Source: CAD feature listing. Evaluate the final solid. Frame: model axes, mm. Face numbers are marked on the shaded views. A direction names the side the tool comes from. Round coordinates to 2 decimals unless told otherwise and drop trailing zeros. Loops run counter-clockwise (first coordinate to the right, second up) from the corner with the lowest first, then second, coordinate; pieces in that order, holes last.
(1) Section A-A, the plane x = 12.5. Return the cut outline in (y, z).
(2) Section B-B, the plane y = 0. Return the cut outline in (x, z), plus the area to 3 significant figures.
(3) Section C-C, the plane z = 4.5. Return the cut outline in (x, y), plus the area to 3 significant figures.
(4) Set-up query: the marked faces 5 and 6. Return all of +Z, -Z, +X, -X, +Y, -Y with unobstructed straight access to the full face (end or side cutting, diameter ignored); none if empty.
(5) Section D-D, the plane x = 0. Return the cut outline in (y, z), plus the area to 3 significant figures.
(6) First-contact query: pin 1 Ø5 at (x, y) = (-2.5, 2.5) entering from +Z; pin 2 Ø2.5 at (x, y) = (24.5, -1.5) entering from +Z; pin 3 Ø1.9 at (x, y) = (-11.5, 0) entering from -Z. Flat tips, straight axial feed; report the tip coordinate or a pass-through.
(7) Mould query, pull axis X, two halves, no side actions, for the marked faces 1, 2, 3 and 4. Classes: pulls with the +X half, pulls with the -X half, needs draft (parallel to the pull), parting line crosses it, or undercut.
(8) Material intervals for probe 1 along Y at (x, z) = (0, 6.5); probe 2 along Y at (x, z) = (-11.5, 5.25); probe 3 along X at (y, z) = (1.5, 1), sorted ascending.
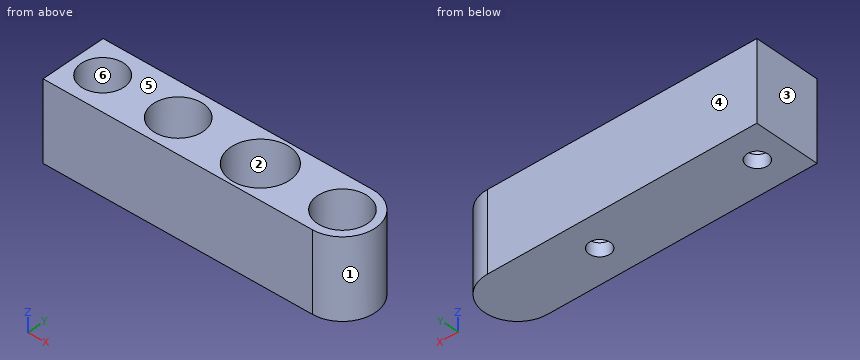
```python
from build123d import *

# Parameters (mm, degrees)
SKETCH_R     = 3.8
SKETCH_R_2   = 4.5
SKETCH_R_3   = 3.25
PAD_DEPTH    = 10
SKETCH001_R  = 1.6
PAD001_DEPTH = 2


with BuildPart() as part:
    # Sketch → Pad (new body)
    with BuildSketch(Plane.XY):
        with BuildLine():
            ThreePointArc((25, -5), (30, 0), (25, 5))
            Line((0, 5), (25, 5))
            Line((0, 5), (-16, 5))
            Line((-16, 5), (-16, -5))
            Line((-16, -5), (0, -5))
            Line((0, -5), (25, -5))
        make_face()
        Circle(SKETCH_R, mode=Mode.SUBTRACT)
        with Locations((25, 0)):
            Circle(SKETCH_R, mode=Mode.SUBTRACT)
        with Locations((12.5, 0)):
            Circle(SKETCH_R_2, mode=Mode.SUBTRACT)
        with Locations((-11.5, 0)):
            Circle(SKETCH_R_3, mode=Mode.SUBTRACT)
    extrude(amount=PAD_DEPTH)

    # Sketch001 (on Face11 of Pad) → Pad001 (join)
    with BuildSketch(Plane(origin=(0, 0, 0), x_dir=(1, 0, 0), z_dir=(0, 0, -1))):
        with BuildLine():
            ThreePointArc((25, -5), (30, 0), (25, 5))
            Line((0, 5), (25, 5))
            Line((0, 5), (-16, 5))
            Line((-16, 5), (-16, -5))
            Line((-16, -5), (0, -5))
            Line((0, -5), (25, -5))
        make_face()
        with Locations((12.5, 0)):
            Circle(SKETCH001_R, mode=Mode.SUBTRACT)
        with Locations((-11.5, 0)):
            Circle(SKETCH001_R, mode=Mode.SUBTRACT)
    extrude(amount=PAD001_DEPTH)


solid = part.part
```
Output values:
1. outline: (-5, -2) - (-1.6, -2) - (-1.6, 0) - (-4.5, 0) - (-4.5, 10) - (-5, 10) - close; (1.6, -2) - (5, -2) - (5, 10) - (4.5, 10) - (4.5, 0) - (1.6, 0) - close
2. outline: (-16, -2) - (-13.1, -2) - (-13.1, 0) - (-14.75, 0) - (-14.75, 10) - (-16, 10) - close; (-9.9, -2) - (10.9, -2) - (10.9, 0) - (8, 0) - (8, 10) - (3.8, 10) - (3.8, 0) - (-3.8, 0) - (-3.8, 10) - (-8.25, 10) - (-8.25, 0) - (-9.9, 0) - close; (14.1, -2) - (30, -2) - (30, 10) - (28.8, 10) - (28.8, 0) - (21.2, 0) - (21.2, 10) - (17, 10) - (17, 0) - (14.1, 0) - close
2. area: 232 mm2
3. outline: (-16, -5) - (25, -5) arc R5 ccw to (25, 5) - (-16, 5) - close; hole circle Ø6.5 at (-11.5, 0); hole circle Ø7.6 at (0, 0); hole circle Ø9 at (12.5, 0); hole circle Ø7.6 at (25, 0)
3. area: 262 mm2
4. face 5: +Z, +X, -X, +Y, -Y
4. face 6: +Z
5. outline: (-5, -2) - (5, -2) - (5, 10) - (3.8, 10) - (3.8, 0) - (-3.8, 0) - (-3.8, 10) - (-5, 10) - close
5. area: 44.0 mm2
6. pin 1: stops at z = 10
6. pin 2: stops at z = 0
6. pin 3: passes through
7. face 1: pulls with the +X half
7. face 2: undercut
7. face 3: pulls with the -X half
7. face 4: needs draft
8. probe 1: y = -5 to -3.8, 3.8 to 5
8. probe 2: y = -5 to -3.25, 3.25 to 5
8. probe 3: x = -16 to -14.38, -8.62 to -3.49, 3.49 to 8.26, 16.74 to 21.51, 28.49 to 29.77
